```python
from build123d import *

# Parameters (mm, degrees)
PAD_DEPTH = 1.8


with BuildPart() as part:
    # Sketch → Pad (new body)
    with BuildSketch(Plane.XZ):
        with BuildLine():
            ThreePointArc((1.59424, 1.405), (-2.125, 0), (1.59424, -1.405))
            Line((3, -1.405), (1.59424, -1.405))
            Line((3, -1.405), (3, -4.125))
            Line((3, -4.125), (0, -4.125))
            ThreePointArc((0, 4.125), (-4.125, 0), (0, -4.125))
            Line((0, 4.125), (3, 4.125))
            Line((3, 4.125), (3, 1.405))
            Line((1.59424, 1.405), (3, 1.405))
        make_face()
    extrude(amount=PAD_DEPTH)


solid = part.part
```
Source: CAD feature listing. Evaluate the final solid. Frame: model axes, mm. A direction names the side the tool comes from. Round coordinates to 2 decimals unless told otherwise and drop trailing zeros. Loops run counter-clockwise (first coordinate to the right, second up) from the corner with the lowest first, then second, coordinate; pieces in that order, holes last.
(1) Section query A-A (y = -0.9). Output: boundary loops of the cut face in (x, z) (3 decimals), and give its area (3 significant figures).
From the geometry:
outline: (0, -4.125) - (3, -4.125) - (3, -1.405) - (1.594, -1.405) arc R2.125 cw (long way) to (1.594, 1.405) - (3, 1.405) - (3, 4.125) - (0, 4.125) arc R4.125 ccw to start
area: 34.4 mm2
(2) Section query D-D (z = 0). Output: boundary loops of the cut face in (x, y) (3 decimals).
From the geometry:
outline: (-4.125, -1.8) - (-2.125, -1.8) - (-2.125, 0) - (-4.125, 0) - close
(3) Contact query for a flat-ended pin moving along its axis: pin 1 Ø3.5 at (x, z) = (0, 0) entering from -Y. Output: stop coordinate, or through.
From the geometry:
pin 1: passes through
(4) Section query B-B (x = 1.5). Output: boundary loops of the cut face in (y, z) (3 decimals), and give its area (3 significant figures).
From the geometry:
outline: (-1.8, -4.125) - (0, -4.125) - (0, -1.505) - (-1.8, -1.505) - close; (-1.8, 1.505) - (0, 1.505) - (0, 4.125) - (-1.8, 4.125) - close
area: 9.43 mm2
(5) Section query C-C (x = 0.5). Output: boundary loops of the cut face in (y, z) (3 decimals).
From the geometry:
outline: (-1.8, -4.125) - (0, -4.125) - (0, -2.065) - (-1.8, -2.065) - close; (-1.8, 2.065) - (0, 2.065) - (0, 4.125) - (-1.8, 4.125) - close
(6) Pull-direction query (X, two-part tool) for faces 3 (the cylindrical face through (-2.124, -0.887, 0.072)), 4 (the flat face through (3, -1, -3)), 5 (the flat face through (2, -1, 1.405)); classes: +X half, -X half, draft (parallel to the pull), parting line (faces both ways), or undercut.
From the geometry:
face 3: undercut
face 4: +X half
face 5: draft
(7) Material intervals for probe 1 along Z at (x, y) = (2.25, -1.4) (3 decimals); probe 2 along Z at (x, y) = (0, -0.95) (3 decimals); probe 3 along X at (y, z) = (-0.1, -1.5), sorted ascending.
From the geometry:
probe 1: z = -4.125 to -1.405, 1.405 to 4.125
probe 2: z = -4.125 to -2.125, 2.125 to 4.125
probe 3: x = -3.84 to -1.51, 1.51 to 3
(8) Access query for faces 1 (the flat face through (-2.1, -1.8, 1)), 2 (the flat face through (2, -1, -1.405)). Directions: +Z, -Z, +X, -X, +Y, -Y. A direction counts if a zero-diameter tool reaches every point of the face in a straight line with its end or side. Return the directions, or none.
From the geometry:
face 1: +Z, -Z, +X, -X, -Y
face 2: +X, +Y, -Y
